Autodesk Inventor part; units mm, degrees
ref_plane "YZ Plane" through (0, 0, 0) normal (1, 0, 0) x (0, 1, 0)
ref_plane "XZ Plane" through (0, 0, 0) normal (0, 1, 0) x (-1, 0, 0)
ref_plane "XY Plane" through (0, 0, 0) normal (0, 0, 1) x (1, 0, 0)
sketch "Sketch1" plane through (0, 0, 0) normal (1, 0, 0) x (0, 1, 0)
  circle A0 centre (0, 0) radius 9.5
  line L0 (0, 9.5) -> (0, 19.5)
  line L1 (0, 19.5) -> (-25, 19.5)
  line L2 (0, -9.5) -> (0, -19.5)
  line L3 (0, -19.5) -> (-25, -19.5)
  line L4 (-25, -19.5) -> (-25, 19.5)
  dimension "d0" = 19
  dimension "d1" = 10
  dimension "d2" = 25
  dimension "d3" = 10
extrude "Extrusion1" add sketch "Sketch1" along normal blind 20 contours A0 L2 L3 L4 L1 L0
sketch "Sketch2" plane through (0, 0, 19.5) normal (0, 1, 0) x (1, 0, 0)
  line L0 (0, 0) -> (0, 5)
  line L1 (0, 0) -> (0, 39)
  line L2 (0, 5) -> (10, 5)
  line L3 (20, 0) -> (20, 39)
  circle A0 centre (10, 5) radius 2.5
  point P0 (0, 19.5)
  dimension "d6" = 5
  dimension "d7" = 10
  dimension "d8" = 5
extrude "Extrusion2" cut sketch "Sketch2" against normal through all
thread "Thread1"
mirror "Mirror2" about plane through (0, 0, 0) normal (0, 0, 1) of "Extrusion2"
properties part number "Clamp" material "Steel, Mild"
Can you work these out from the model? Positions are in its coordinate system, mm. Give positions to 0.01 mm unless a question says otherwise; leave off trailing zeros. Loops run counter-clockwise (first coordinate to the right, second up) from the corner with the lowest first, then second, coordinate; pieces in that order, holes last. Notation, with made-up numbers: (19.25, 37.5) -> (63.25, 37.5) arc R18 ccw to (63.25, 53.5) -> close; hole circle Ø6 at (-12.75, 45.5). An arc over 180 degrees is marked (long way). Return JSON: item names as keys, results as strings.
Q1. I want a section at B-B, the plane y = -3.75. List the corners of the cut face in (x, z) for me.
Checks:
{"outline": "(0, -19.5) -> (20, -19.5) -> (20, -8.73) -> (0, -8.73) -> close; (0, 8.73) -> (20, 8.73) -> (20, 19.5) -> (0, 19.5) -> close; hole circle Ø5 at (10, -14.5); hole circle Ø5 at (10, 14.5)"}
Q2. I want a section at D-D, the plane y = -13. List the corners of the cut face in (x, z) for me, then the cut area to 3 significant figures.
Checks:
{"outline": "(0, -19.5) -> (20, -19.5) -> (20, 19.5) -> (0, 19.5) -> close; hole circle Ø5 at (10, -14.5); hole circle Ø5 at (10, 14.5)", "area": "741 mm2"}
Q3. I need wall thicknesses on probe 1 along Z at (x, y) = (10, -16.5); probe 2 along Z at (x, y) = (9.25, -4); probe 3 along Z at (x, y) = (12, -23.25). Which ranges of each line are inside material? Lowest first, please.
Checks:
{"probe 1": "z = -19.5 to -17, -12 to 12, 17 to 19.5", "probe 2": "z = -19.5 to -16.88, -12.12 to -8.62, 8.62 to 12.12, 16.88 to 19.5", "probe 3": "z = -19.5 to -16, -13 to 13, 16 to 19.5"}
Q4. For pin 1 Ø1 at (x, z) = (14.5, -4) entering from +Y; pin 2 Ø1 at (y, z) = (-8, -3) entering from +X, each with a flat end and sliding along its axis, tell me the tip position at first contact or that it passes through.
Checks:
{"pin 1": "stops at y = -8.37", "pin 2": "passes through"}
Q5. We'd pull the mould along Z, two halves only. Please class faces 1 (the face through (9.46, -12.32, 16.94)), 2 (the face through (9.86, -9.498, -0.209)), 3 (the face through (7.6, 0, -13.3)), 4 (the face through (10, -12, 19.5)): released by +Z, released by -Z, zero draft, split by the parting line, or undercut.
Checks:
{"face 1": "undercut", "face 2": "undercut", "face 3": "zero draft", "face 4": "released by +Z"}
Q6. I want a section at C-C, the plane z = -13. List the corners of the cut face in (x, y) for me.
Checks:
{"outline": "(0, -25) -> (8, -25) -> (8, 0) -> (0, 0) -> close; (12, -25) -> (20, -25) -> (20, 0) -> (12, 0) -> close"}
Q7. I want a section at A-A, the plane x = 10. List the corners of the cut face in (y, z) for me.
Checks:
{"outline": "(-25, -19.5) -> (0, -19.5) -> (0, -17) -> (-25, -17) -> close; (-25, -12) -> (0, -12) -> (0, -9.5) arc R9.5 cw to (0, 9.5) -> (0, 12) -> (-25, 12) -> close; (-25, 17) -> (0, 17) -> (0, 19.5) -> (-25, 19.5) -> close"}
